CAD build for the part. Positions are in the model's coordinates, mm. A direction names the side the tool comes from. Coordinates: 2 decimals unless noted, no trailing zeros. Write each loop counter-clockwise with the first axis right and the second up, starting at its lowest first coordinate (ties: lowest second). Pieces come first, ordered by that corner, then holes. Notation, with made-up numbers: (65.25, -24.5) - (78.25, -24.5) arc R22 ccw to (78.25, -15.5) - close; hole circle Ø7 at (72.5, 33.5). An arc over 180 degrees is marked (long way). Answer in a Markdown table with one row per item. Add a question column.
Q1. Band-saw the part on A-A (z = 40.5). List the corners of the cut face in (x, y).
Q2. Pin check, flat tip, straight feed: pin 1 (2 mm diameter, centred on x = 40, y = 73, fed in from +Z). Stop position of the tip, or through.
Q3. 3-axis set-ups, long thin cutter, end or side, ignore diameter. For faces 5 (the flat face through (84, 5, 20)), 6 (the cylindrical face through (164.98, 80.75, 27.08)), 7 (the flat face through (84, 3, 35)): which of +Z, -Z, +X, -X, +Y, -Y reach the whole face in a straight line?
Q4. Band-saw the part on B-B (y = 109). List the corners of the cut face in (x, z), and give its area (3 significant figures).
Q5. Two-plate mould, pull along X, no slides. Class faces 1 (the flat face through (84, 84, 5)), 2 (the flat face through (84, 84, 0)), 3 (the cylindrical face through (10.44, 124.82, 18.68)), 4 (the flat face through (0, 82, 21)): +X half, -X half, draft (parallel to the pull), parting line (faces both ways), or undercut.
Q6. Drill centre lines: line 1 along X through (y, z) = (34, 38); line 2 along Y through (x, z) = (40, 33); line 3 along Y through (x, z) = (147.5, 41). Where is each one in solid material? Low to high. Write a range as from..to.
```python
from build123d import *

# Parameters (mm, degrees)
SKETCH1_W               = 170.47
SKETCH1_H               = 165.71
BOSS_EXTRUDE1_DEPTH     = 5
SKETCH2_W               = 170.47
SKETCH2_H               = 165.71
SKETCH2_W_2             = 160.47
SKETCH2_H_2             = 155.71
BOSS_EXTRUDE2_DEPTH     = 38
SKETCH3_W               = 160.47
SKETCH3_H               = 5
CUT_EXTRUDE1_DEPTH      = 8
SKETCH5_R               = 5.5
BOSS_EXTRUDE3_DEPTH     = 1
SKETCH6_R               = 4.5
BOSS_EXTRUDE4_DEPTH     = 9
LPATTERN1_COUNT         = 3
LPATTERN1_PITCH         = 38.9275
MIRROR1_COPY_1_SKETCH_R = 5.5
MIRROR1_COPY_1_DEPTH    = 1
MIRROR1_COPY_2_SKETCH_R = 5.5
MIRROR1_COPY_2_DEPTH    = 1
MIRROR1_COPY_3_SKETCH_R = 4.5
MIRROR1_COPY_3_DEPTH    = 9
MIRROR1_COPY_4_SKETCH_R = 4.5
MIRROR1_COPY_4_DEPTH    = 9


with BuildPart() as part:
    # Sketch1 → Boss-Extrude1 (new body)
    with BuildSketch(Plane.XY):
        with Locations((85.235, 82.855)):
            Rectangle(SKETCH1_W, SKETCH1_H)
    extrude(amount=BOSS_EXTRUDE1_DEPTH)

    # Sketch2 → Boss-Extrude2 (add)
    with BuildSketch(Plane.XY.offset(5)):
        with Locations((85.235, 82.855)):
            Rectangle(SKETCH2_W, SKETCH2_H)
        with Locations((85.235, 82.855)):
            Rectangle(SKETCH2_W_2, SKETCH2_H_2, mode=Mode.SUBTRACT)
    extrude(amount=BOSS_EXTRUDE2_DEPTH)

    # Sketch3 → Cut-Extrude1 (cut)
    with BuildSketch(Plane.XY.offset(43)):
        with Locations((85.235, 2.5)):
            Rectangle(SKETCH3_W, SKETCH3_H)
    extrude(amount=-CUT_EXTRUDE1_DEPTH, mode=Mode.SUBTRACT)

    # Sketch5 → Boss-Extrude3 (add)
    with BuildSketch(Plane.ZY.offset(-165.47)):
        with Locations((22, 121.7825)):
            Circle(SKETCH5_R)
    boss_extrude3 = extrude(amount=BOSS_EXTRUDE3_DEPTH)

    # Sketch6 → Boss-Extrude4 (add)
    with BuildSketch(Plane.ZY.offset(-164.47)):
        with Locations((22, 121.7825)):
            Circle(SKETCH6_R)
    boss_extrude4 = extrude(amount=BOSS_EXTRUDE4_DEPTH)

    # LPattern1: Boss-Extrude3, Boss-Extrude4 ×3
    with Locations(*[(0, -i * LPATTERN1_PITCH, 0) for i in range(1, LPATTERN1_COUNT)]):
        add(boss_extrude3)
        add(boss_extrude4)

    # Mirror1: Boss-Extrude3, Boss-Extrude4 across plane
    add(boss_extrude3.mirror(Plane.ZY.offset(-85.235)))
    add(boss_extrude4.mirror(Plane.ZY.offset(-85.235)))

    # Mirror1 copy 1 sketch → Mirror1 copy 1 (add)
    with BuildSketch(Plane(origin=(5, -38.9275, 0), x_dir=(0, 0, 1), z_dir=(1, 0, 0))):
        with Locations((22, -121.7825)):
            Circle(MIRROR1_COPY_1_SKETCH_R)
    extrude(amount=MIRROR1_COPY_1_DEPTH)

    # Mirror1 copy 2 sketch → Mirror1 copy 2 (add)
    with BuildSketch(Plane(origin=(5, -77.855, 0), x_dir=(0, 0, 1), z_dir=(1, 0, 0))):
        with Locations((22, -121.7825)):
            Circle(MIRROR1_COPY_2_SKETCH_R)
    extrude(amount=MIRROR1_COPY_2_DEPTH)

    # Mirror1 copy 3 sketch → Mirror1 copy 3 (add)
    with BuildSketch(Plane(origin=(6, -38.9275, 0), x_dir=(0, 0, 1), z_dir=(1, 0, 0))):
        with Locations((22, -121.7825)):
            Circle(MIRROR1_COPY_3_SKETCH_R)
    extrude(amount=MIRROR1_COPY_3_DEPTH)

    # Mirror1 copy 4 sketch → Mirror1 copy 4 (add)
    with BuildSketch(Plane(origin=(6, -77.855, 0), x_dir=(0, 0, 1), z_dir=(1, 0, 0))):
        with Locations((22, -121.7825)):
            Circle(MIRROR1_COPY_4_SKETCH_R)
    extrude(amount=MIRROR1_COPY_4_DEPTH)


solid = part.part
```
Checked values:
| question | item | result |
|---|---|---|
| 1 | outline | (0, 0) - (5, 0) - (5, 160.71) - (165.47, 160.71) - (165.47, 0) - (170.47, 0) - (170.47, 165.71) - (0, 165.71) - close |
| 2 | pin 1 | stops at z = 5 |
| 3 | face 5 | +Z |
| 3 | face 6 | none |
| 3 | face 7 | +Z, -Y |
| 4 | outline | (0, 0) - (170.47, 0) - (170.47, 43) - (165.47, 43) - (165.47, 5) - (5, 5) - (5, 43) - (0, 43) - close |
| 4 | area | 1,230 mm² |
| 5 | face 1 | undercut |
| 5 | face 2 | draft |
| 5 | face 3 | undercut |
| 5 | face 4 | -X half |
| 6 | line 1 | x = 0..5, 165.47..170.47 |
| 6 | line 2 | y = 0..5, 160.71..165.71 |
| 6 | line 3 | y = 160.71..165.71 |
